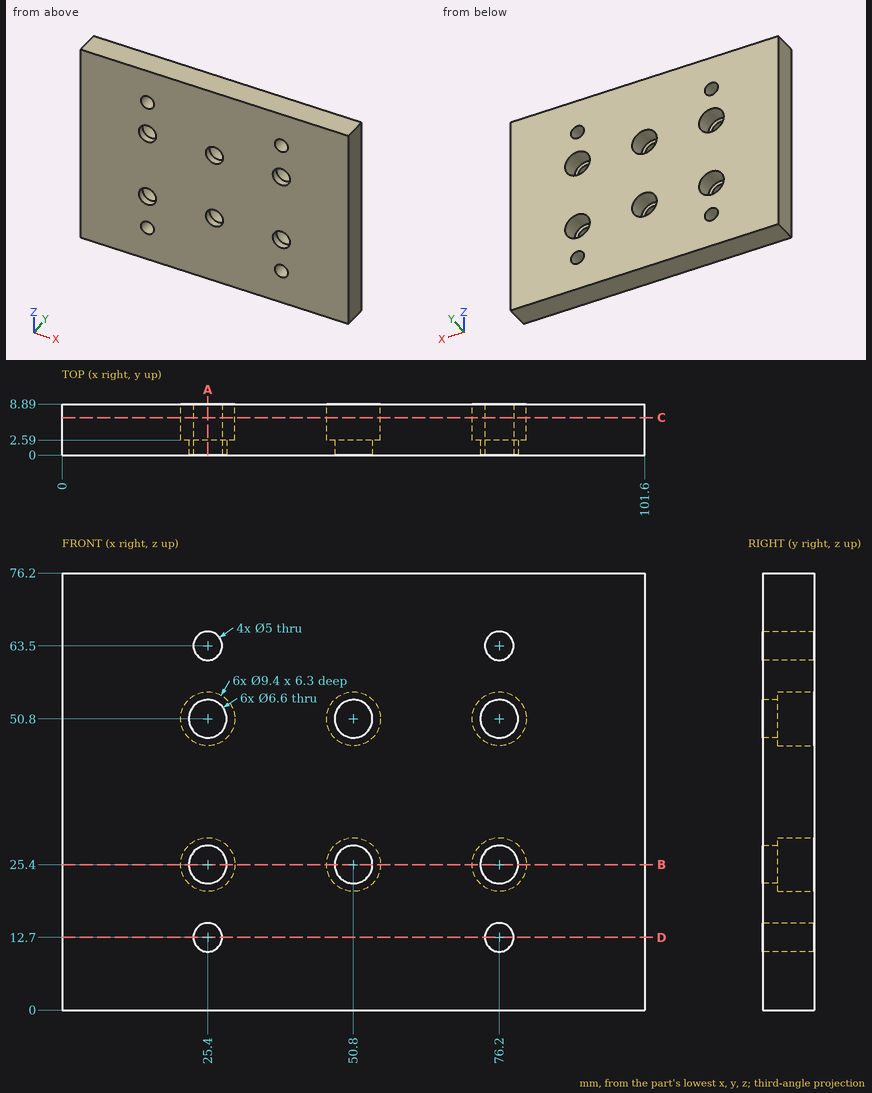
Here's the drawing with two shaded views (mm, measured from the low corner). I have some questions. Coordinates: 2 decimals unless noted, no trailing zeros. Write each loop counter-clockwise with the first axis right and the second up, starting at its lowest first coordinate (ties: lowest second). Pieces come first, ordered by that corner, then holes.
Item 1: If I drill on line 1 (Z direction, x = 76.2, y = 6.5); line 2 (X direction, y = 6.75, z = 63.5); line 3 (X direction, y = 1.15, z = 50.8), over which ranges is the centre line in solid material (lowest first)?
Item 2: I want a section at C-C on y = 6.5. Count the separate pieces of the cut face and the enclosed holes in it, and give its area (3 significant figures).
Item 3: I want a section at A-A on x = 25.4. Write out the boundary of the cut face in (y, z), and give its area (3 significant figures).
Item 4: Will these pins go through, and if not, where does the flat tip stop? pin 1 (8.5 mm diameter, centred on x = 76.2, z = 50.8, fed in from +Y); pin 2 (4 mm diameter, centred on x = 76.2, z = 63.5, fed in from +Y).
Item 5: I want a section at D-D on z = 12.7. Write out the boundary of the cut face in (x, y), and give its area (3 significant figures).
Item 6: I want a section at B-B on z = 25.4. Write out the boundary of the cut face in (x, y).
Findings below:
1. line 1: z = 0 to 10.2, 15.2 to 20.7, 30.1 to 46.1, 55.5 to 61, 66 to 76.2
1. line 2: x = 0 to 22.9, 27.9 to 73.7, 78.7 to 101.6
1. line 3: x = 0 to 22.1, 28.7 to 47.5, 54.1 to 72.9, 79.5 to 101.6
2. separate pieces: 1
2. enclosed holes: 10
2. area: 7,250 mm2
3. outline: (0, 0) - (8.89, 0) - (8.89, 10.2) - (0, 10.2) - close; (0, 15.2) - (8.89, 15.2) - (8.89, 20.7) - (2.59, 20.7) - (2.59, 22.1) - (0, 22.1) - close; (0, 28.7) - (2.59, 28.7) - (2.59, 30.1) - (8.89, 30.1) - (8.89, 46.1) - (2.59, 46.1) - (2.59, 47.5) - (0, 47.5) - close; (0, 54.1) - (2.59, 54.1) - (2.59, 55.5) - (8.89, 55.5) - (8.89, 61) - (0, 61) - close; (0, 66) - (8.89, 66) - (8.89, 76.2) - (0, 76.2) - close
3. area: 436 mm2
4. pin 1: stops at y = 2.59
4. pin 2: passes through
5. outline: (0, 0) - (22.9, 0) - (22.9, 8.89) - (0, 8.89) - close; (27.9, 0) - (73.7, 0) - (73.7, 8.89) - (27.9, 8.89) - close; (78.7, 0) - (101.6, 0) - (101.6, 8.89) - (78.7, 8.89) - close
5. area: 814 mm2
6. outline: (0, 0) - (22.1, 0) - (22.1, 2.59) - (20.7, 2.59) - (20.7, 8.89) - (0, 8.89) - close; (28.7, 0) - (47.5, 0) - (47.5, 2.59) - (46.1, 2.59) - (46.1, 8.89) - (30.1, 8.89) - (30.1, 2.59) - (28.7, 2.59) - close; (54.1, 0) - (72.9, 0) - (72.9, 2.59) - (71.5, 2.59) - (71.5, 8.89) - (55.5, 8.89) - (55.5, 2.59) - (54.1, 2.59) - close; (79.5, 0) - (101.6, 0) - (101.6, 8.89) - (80.9, 8.89) - (80.9, 2.59) - (79.5, 2.59) - close
